```python
from build123d import *

# Parameters (mm, degrees)
CYLINDER_R     = 25
CYLINDER_DEPTH = 1000
CUBE_W         = 100
CUBE_H         = 100
CUBE_DEPTH     = 100


with BuildPart() as cylinder:
    # cylinder → cylinder (new body)
    with BuildSketch(Plane.XY.offset(100)):
        Circle(CYLINDER_R)
    extrude(amount=CYLINDER_DEPTH)


with BuildPart() as sphere:
    # sphere → sphere (revolve)
    with BuildSketch(Plane(origin=(0, 0, 1100), x_dir=(1, 0, 0), z_dir=(0, -1, 0))):
        with BuildLine():
            ThreePointArc((0, -50), (50, 0), (0, 50))
            Line((0, 50), (0, -50))
        make_face()
    revolve(axis=Axis((0, 0, 1100), (0, 0, 1)))


with BuildPart() as union:
    # cube → cube (new body)
    with BuildSketch(Plane(origin=(-50, -50, 0), x_dir=(1, 0, 0), z_dir=(0, 0, 1))):
        with Locations((50, 50)):
            Rectangle(CUBE_W, CUBE_H)
    extrude(amount=CUBE_DEPTH)

    # union: union cylinder, sphere
    add(cylinder.part)
    add(sphere.part)


solid = union.part
```
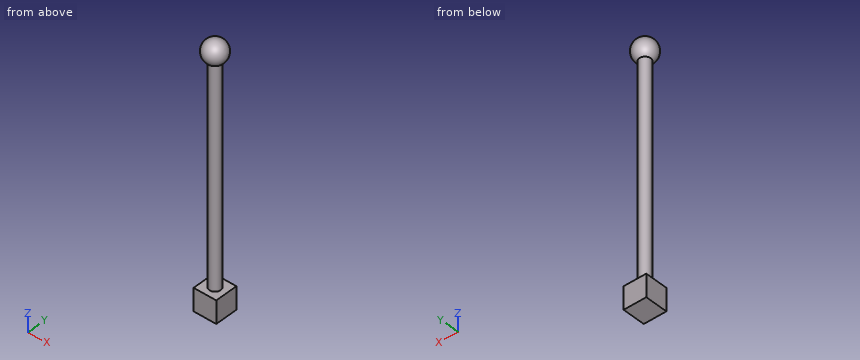
The model under review builds one solid part; all positions refer to its coordinate system, in mm. Round coordinates to 2 decimals unless told otherwise and drop trailing zeros. Loops run counter-clockwise (first coordinate to the right, second up) from the corner with the lowest first, then second, coordinate; pieces in that order, holes last. Notation, with made-up numbers: (59.5, -23) - (76.5, -23) arc R33 ccw to (76.5, 13) - close; hole circle Ø3 at (27.25, 20.25). An arc over 180 degrees is marked (long way). Use a Markdown table: item, result. Add a question column.
Q1. Insertion check: pin 1 Ø3 at (y, z) = (-14.5, 514.5) entering from +X; pin 2 Ø1 at (x, y) = (39, -35) entering from -Z; pin 3 Ø1 at (x, y) = (-27.5, 35.5) entering from +Z; pin 4 Ø5 at (x, z) = (-6, 598) entering from -Y. Each pin has a flat end and moves straight along its axis. Give the tip position at first contact, or say it passes through.
Q2. For probe 1 along Z at (x, y) = (26, 19); probe 2 along Z at (x, y) = (24.5, 21.5); probe 3 along X at (y, z) = (2, 893), list the stretches that pass through material, from the lowest coordinate up.
Q3. Add section C-C (z = 352.5). State the section outline as (x, y) points.
Q4. Add section B-B (x = -15). State the section outline as (y, z) points.
Q5. Add section A-A (y = -40). State the section outline as (x, z) points, plus the area to 3 significant figures.
Q6. Add section D-D (y = 36.5). State the section outline as (x, z) points.
Worked answers:
| question | item | result |
|---|---|---|
| 1 | pin 1 | x = 21.35 |
| 1 | pin 2 | z = 0 |
| 1 | pin 3 | z = 1122.98 |
| 1 | pin 4 | y = -24.75 |
| 2 | probe 1 | 0 to 100, 1061.75 to 1138.25 |
| 2 | probe 2 | 0 to 100, 1062.09 to 1137.91 |
| 2 | probe 3 | -24.92 to 24.92 |
| 3 | outline | circle Ø50 at (0, 0) |
| 4 | outline | (-50, 0) - (50, 0) - (50, 100) - (20, 100) - (20, 1056.7) arc R47.7 ccw (long way) to (-20, 1056.7) - (-20, 100) - (-50, 100) - close |
| 5 | outline | (-50, 0) - (50, 0) - (50, 100) - (-50, 100) - close; circle Ø60 at (0, 1100) |
| 5 | area | 12,800 mm² |
| 6 | outline | (-50, 0) - (50, 0) - (50, 100) - (-50, 100) - close; circle Ø68.34 at (0, 1100) |
